```python
from build123d import *

# Parameters (mm, degrees)
SKETCH_1_R      = 1.5
EXTRUDE_1_DEPTH = 4


with BuildPart() as part:
    # Эскиз1 → Бобышка-Вытянуть1 (new body)
    with BuildSketch(Plane(origin=(0, 0, 0), x_dir=(1, 0, 0), z_dir=(0, 1, 0))):
        with BuildLine():
            Line((-50, 0), (-43, 0))
            Line((-43, 0), (-39, 0))
            Line((-39, 0), (-38, 1))
            Line((-38, 1), (-35, -2))
            Line((-35, -2), (-33, 0))
            Line((-33, 0), (-32, 1))
            Line((-32, 1), (-29, -2))
            Line((-29, -2), (-27, 0))
            Line((-27, 0), (-26, 1))
            Line((-26, 1), (-23, -2))
            Line((-23, -2), (-21, 0))
            Line((-21, 0), (-20, 1))
            Line((-20, 1), (-17, -2))
            Line((-17, -2), (-15, 0))
            Line((-15, 0), (-14, 1))
            Line((-14, 1), (-11, -2))
            Line((-11, -2), (-9, 0))
            Line((-9, 0), (-8, 1))
            Line((-8, 1), (-5, -2))
            Line((-5, -2), (-3, 0))
            Line((-3, 0), (-2, 1))
            Line((-2, 1), (1, -2))
            Line((1, -2), (3, 0))
            Line((3, 0), (4, 1))
            Line((4, 1), (7, -2))
            Line((7, -2), (9, 0))
            Line((9, 0), (10, 1))
            Line((10, 1), (13, -2))
            Line((13, -2), (15, 0))
            Line((15, 0), (16, 1))
            Line((16, 1), (19, -2))
            Line((19, -2), (21, 0))
            Line((21, 0), (22, 1))
            Line((22, 1), (25, -2))
            Line((25, -2), (27, 0))
            Line((27, 0), (28, 1))
            Line((28, 1), (31, -2))
            Line((31, -2), (33, 0))
            Line((33, 0), (34, 1))
            Line((34, 1), (37, -2))
            Line((37, -2), (39, 0))
            Line((39, 0), (43, 0))
            Line((43, 0), (50, 0))
            add(Edge.make_bspline(
                [(50, 0), (50, 9.148701546), (38.189799805, 16.136443156)],
                knots=[6.270008338, 6.270008338, 6.270008338, 6.984807717, 6.984807717, 6.984807717], degree=2, weights=[0.818101322, 0.849400917, 1]))
            Line((38.189799805, 16.136443156), (34.912704057, 10.507753014))
            add(Edge.make_bspline(
                [(42.090540855, 3.682445167), (40.227847319, 7.413208709), (34.912704057, 10.507753014)],
                knots=[0.206034906, 0.206034906, 0.206034906, 0.623356981, 0.623356981, 0.623356981], degree=2, weights=[1, 0.978309158, 1]))
            Line((42.090540855, 3.682445167), (39, 1))
            Line((39, 1), (37, -1))
            Line((37, -1), (34, 2))
            Line((34, 2), (33, 1))
            Line((33, 1), (31, -1))
            Line((31, -1), (28, 2))
            Line((28, 2), (27, 1))
            Line((27, 1), (25, -1))
            Line((25, -1), (22, 2))
            Line((22, 2), (21, 1))
            Line((21, 1), (19, -1))
            Line((19, -1), (16, 2))
            Line((16, 2), (15, 1))
            Line((15, 1), (13, -1))
            Line((13, -1), (10, 2))
            Line((10, 2), (9, 1))
            Line((9, 1), (7, -1))
            Line((7, -1), (4, 2))
            Line((4, 2), (3, 1))
            Line((3, 1), (1, -1))
            Line((1, -1), (-2, 2))
            Line((-2, 2), (-3, 1))
            Line((-3, 1), (-5, -1))
            Line((-5, -1), (-8, 2))
            Line((-8, 2), (-9, 1))
            Line((-9, 1), (-11, -1))
            Line((-11, -1), (-14, 2))
            Line((-14, 2), (-15, 1))
            Line((-15, 1), (-17, -1))
            Line((-17, -1), (-20, 2))
            Line((-20, 2), (-21, 1))
            Line((-21, 1), (-23, -1))
            Line((-23, -1), (-26, 2))
            Line((-26, 2), (-27, 1))
            Line((-27, 1), (-29, -1))
            Line((-29, -1), (-32, 2))
            Line((-32, 2), (-33, 1))
            Line((-33, 1), (-35, -1))
            Line((-35, -1), (-38, 2))
            Line((-38, 2), (-39, 1))
            Line((-39, 1), (-42.090540855, 3.682445167))
            add(Edge.make_bspline(
                [(-34.912704057, 10.507753014), (-40.227846573, 7.413208572), (-42.090540855, 3.682445167)],
                knots=[5.659828256, 5.659828256, 5.659828256, 6.077150244, 6.077150244, 6.077150244], degree=2, weights=[1, 0.978309167, 1]))
            Line((-34.912704057, 10.507753014), (-38.189799805, 16.136443156))
            add(Edge.make_bspline(
                [(-38.189799805, 16.136443156), (-50, 9.148701546), (-50, 0)],
                knots=[2.439970244, 2.439970244, 2.439970244, 3.141592654, 3.141592654, 3.141592654], degree=2, weights=[1, 0.939094243, 1]))
        make_face()
        with Locations(Location((-45.689262056, 3.997292475, 0), (0, 0, 270))):
            Circle(SKETCH_1_R, mode=Mode.SUBTRACT)
        with Locations(Location((-40.232363482, 10.780229305, 0), (0, 0, 270))):
            Circle(SKETCH_1_R, mode=Mode.SUBTRACT)
        with Locations(Location((45.689262056, 3.997292475, 0), (0, 0, 270))):
            Circle(SKETCH_1_R, mode=Mode.SUBTRACT)
        with Locations(Location((40.232363482, 10.780229305, 0), (0, 0, 270))):
            Circle(SKETCH_1_R, mode=Mode.SUBTRACT)
    extrude(amount=EXTRUDE_1_DEPTH)


solid = part.part
```
Could you check a few things on this model? Use its own coordinates, in mm. A direction names the side the tool comes from. Coordinates: 2 decimals unless noted, no trailing zeros. Write each loop counter-clockwise with the first axis right and the second up, starting at its lowest first coordinate (ties: lowest second). Pieces come first, ordered by that corner, then holes. Notation, with made-up numbers: (-25.75, 61) - (14.25, 61) arc R19 cw to (14.25, 85) - close; hole circle Ø4 at (83, -28.75). An arc over 180 degrees is marked (long way). Use a Markdown table: item, result.
Q1. Which directions (+Z, -Z, +X, -X, +Y, -Y) give clear straight access to the entire face, cutting with the end or side of a thin tool? Please do faces 1 (the flat face through (-18, 2, 0)), 2 (the flat face through (-45, 2, 0)), 3 (the flat face through (-4, 2, 1)).
Geometry check:
| item | result |
|---|---|
| face 1 | -Z, +Y, -Y |
| face 2 | +Z, -X, +Y, -Y |
| face 3 | +Z, +Y, -Y |
Q2. Thinking about a two-plate mould opening in Z: for faces 4 (the flat face through (-25, 2, 0)), 5 (the flat face through (-24, 2, 0)), 6 (the flat face through (-36, 2, 0)), which applies, +Z half, -Z half, draft (parallel to the pull), parting line (faces both ways), or undercut?
Geometry check:
| item | result |
|---|---|
| face 4 | +Z half |
| face 5 | -Z half |
| face 6 | undercut |
Q3. Imagine slicing it at A-A (x = 20.5). List the corners of the cut face in (y, z) for me.
Geometry check:
| item | result |
|---|---|
| outline | (0, -0.5) - (4, -0.5) - (4, 0.5) - (0, 0.5) - close |
Q4. I'm going to push flat-ended pins straight in: pin 1 Ø3.5 at (x, z) = (-45.69, -4) entering from +Y; pin 2 Ø1 at (y, z) = (1.5, -4) entering from +X. Where does each tip first touch, or does it pass through?
Geometry check:
| item | result |
|---|---|
| pin 1 | stops at y = 4 |
| pin 2 | stops at x = 49.51 |
Q5. Imagine slicing it at B-B (y = 0.9). Count the separate pieces of the cut face and the enclosed holes in it, and give its area (3 significant figures).
Geometry check:
| item | result |
|---|---|
| separate pieces | 1 |
| enclosed holes | 4 |
| area | 301 mm2 |
Q6. Please list where these lines run through material, in increasing order: L1, parallel to X at y = 1.7, z = -9.5; L2, parallel to X at y = 3, z = -11.5; L3, parallel to Z at x = -11, y = 3.25.
Geometry check:
| item | result |
|---|---|
| L1 | x = -46.25 to -41.01, -39.45 to -36.52, 36.52 to 39.45, 41.01 to 46.25 |
| L2 | x = -44.4 to -41.55, -38.92 to -35.49, 35.49 to 38.92, 41.55 to 44.4 |
| L3 | z = 1 to 2 |
